from build123d import *

# Parameters (mm, degrees)
F2_R = 5
F3_R = 0.7471384798
F5_R = 3.0872818621


# Not quite as in the source:
# - a fillet or chamfer that OpenCascade refuses, or shapes differently, is made with other operations: its cross-section is extruded or revolved along the edge and cut away or added


with BuildPart() as f1:
    # F0 (on Front) → F1 (revolve)
    with BuildSketch(Plane.XZ):
        Polygon((-10.6199271977, 0), (0, 0), (0, 20.5089394003), (-6.1166980304, 20.5089394003), (-7.7893259004, 18.9006421715), (-9.590617381, 18.9649742097), (-10.5555951595, 20.4446054995), (-17.6320988685, 20.3159432858), (-17.6320988685, 19.0936364233), (-10.748591274, 15.3623912483), (-12.7428779379, 7.8355651349), align=None)
    revolve(axis=Axis((0, 0, 10.2544697002), (0, 0, -1)))

    # F2
    f2_edges = [f1.edges().sort_by_distance(p)[0] for p in [
        (6.116698, 0, 20.508939),
    ]]
    fillet(f2_edges, radius=F2_R)

    # F3
    f3_edges = [f1.edges().sort_by_distance(p)[0] for p in [
        (17.632099, 0, 20.315943),
    ]]
    fillet(f3_edges, radius=F3_R)

    # F4: fillet of radius 5 on 1 edges, made by hand

    # F4_s1 → F4_t2 (revolve, cut)
    with BuildSketch(Plane.XZ):
        with BuildLine():
            ThreePointArc((-17.6320943676, 19.5822655038), (-16.9135613616, 18.827647757), (-16.0542267415, 18.2383416946))
            Line((-16.0542267415, 18.2383416946), (-17.6320988685, 19.0936364233))
            ThreePointArc((-17.6320988685, 19.0936364233), (-17.6320988685, 19.3379509636), (-17.6320943676, 19.5822655038))
        make_face()
    revolve(axis=Axis((0, 0, 19.0936364233), (0, 0, -1)), mode=Mode.SUBTRACT)

    # F5
    f5_edges = [f1.edges().sort_by_distance(p)[0] for p in [
        (12.742878, 0, 7.835565),
        (10.619927, 0, 0),
        (-11.681403, 0, 3.917783),
    ]]
    fillet(f5_edges, radius=F5_R)


solid = f1.part
The listing builds one solid part. Answer for the finished solid, in the listing's coordinates (mm). A direction names the side the tool comes from. Give positions to 0.01 mm unless a question says otherwise; leave off trailing zeros. Write each loop counter-clockwise with the first axis right and the second up, starting at its lowest first coordinate (ties: lowest second). Pieces come first, ordered by that corner, then holes. Notation, with made-up numbers: (28.25, 22) -> (33.25, 22) arc R21 cw to (33.25, 30) -> close; hole circle Ø1 at (-6.75, 67.25). An arc over 180 degrees is marked (long way). Use a Markdown table: item, result.
(1) Find the intervals of material crossed by probe 1 along Z at (x, y) = (-5, 6); probe 2 along Z at (x, y) = (-1.5, -14.5); probe 3 along Y at (x, z) = (-9, 5.25), in increasing order. Write a range as from..to.
Return value:
| item | result |
|---|---|
| probe 1 | 0..18.9 |
| probe 2 | 17.44..20.37 |
| probe 3 | -8..8 |
(2) Section B-B, the plane z = 14 is taken. Determine the outline of the cut face in (x, y).
Return value:
| item | result |
|---|---|
| outline | circle Ø22.22 at (0, 0) |
(3) For faces 1 (the flat face through (0, 0, 20.509)), 2 (the conical face through (1.426, 10.859, 20.437)), 3 (the conical face through (1.43, 10.91, 15.5)), determine the directions among +Z, -Z, +X, -X, +Y, -Y from which every point of the face is accessible in a straight line to the end or side of a thin tool.
Return value:
| item | result |
|---|---|
| face 1 | +Z, +X, -X, +Y, -Y |
| face 2 | +Z |
| face 3 | none |
(4) Flat-ended cylindrical pins translate along their axes: P1, Ø1.5, axis at x = 2, z = 8, coming from the +Y side; P2, Ø5, axis at x = -7, z = 14, coming from the +Y side; P3, Ø10, axis at x = 0, z = 12, coming from the -Y side. Find the tip coordinate at first contact, or state that the pin passes through.
Return value:
| item | result |
|---|---|
| P1 | y = 12.57 |
| P2 | y = 10.99 |
| P3 | y = -13.77 |
(5) Section A-A, the plane z = 17.5 is taken. Determine the outline of the cut face in (x, y), then the cut area to 3 significant figures.
Return value:
| item | result |
|---|---|
| outline | circle Ø29.38 at (0, 0) |
| area | 678 mm2 |
